Source: three-view drawing plus pictorial views. Frame: mm from the lowest corner of the part. Coordinates: 2 decimals unless noted, no trailing zeros. Write each loop counter-clockwise with the first axis right and the second up, starting at its lowest first coordinate (ties: lowest second). Pieces come first, ordered by that corner, then holes. Notation, with made-up numbers: (-33, -36) - (13, -36) arc R4 ccw to (13, -31) - close; hole circle Ø7 at (29, 72). An arc over 180 degrees is marked (long way). Put each result on its own line as item: value. Start each with the question number.
1. Pin query (flat end, axial travel): pin 1 (3 mm diameter, centred on y = 26.5, z = 4, fed in from -X); pin 2 (7 mm diameter, centred on x = 10, y = 10, fed in from -Z). Return the tip coordinate at first contact, or that it passes through.
2. Cut plane A-A, the plane y = 10. Return loops of the section in (x, z), and give its area (3 significant figures).
3. Cut plane D-D, the plane y = 25. Return loops of the section in (x, z).
4. Cut plane C-C, the plane x = 35. Return loops of the section in (y, z).
5. Pull-direction query (Y, two-part tool) for the marked faces 1, 2 and 3; classes: released by +Y, released by -Y, zero draft, split by the parting line, or undercut.
6. Cut plane B-B, the plane z = 5.25. Return loops of the section in (x, y).
7. Line query: line 1 (Y direction, x = 35, z = 3.8); line 2 (X direction, y = 7.5, z = 2); line 3 (Y direction, x = 35, z = 3.7). Output: solid intervals per line, ascending.
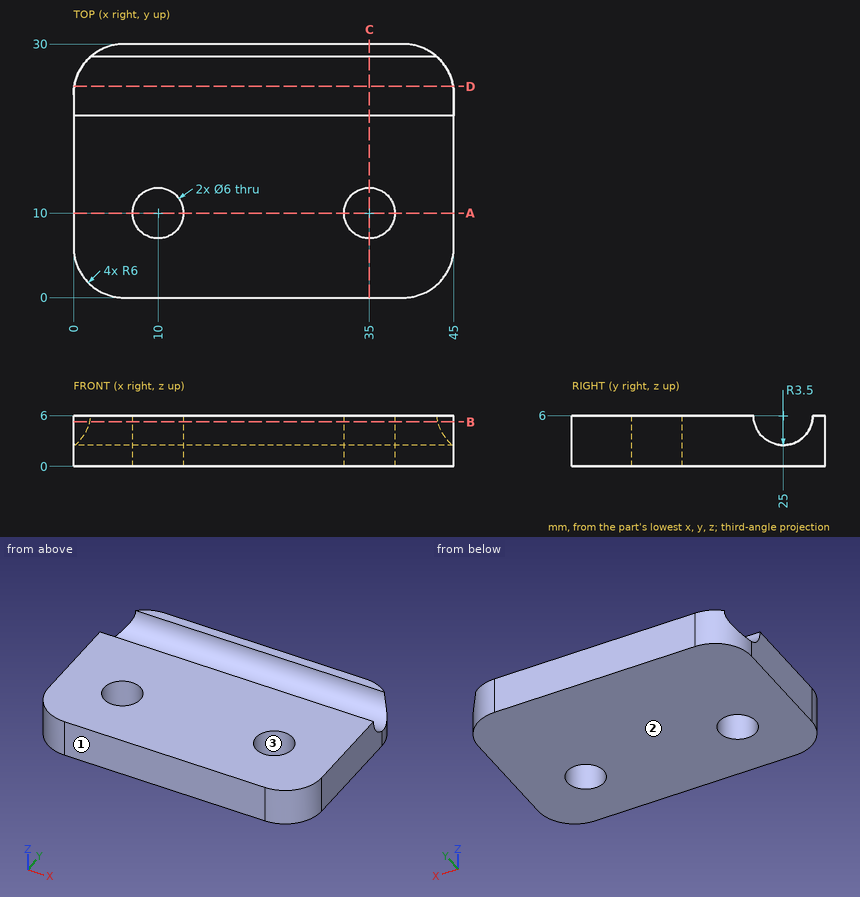
Report:
1. pin 1: stops at x = 0.31
1. pin 2: stops at z = 0
2. outline: (0, 0) - (7, 0) - (7, 6) - (0, 6) - close; (13, 0) - (32, 0) - (32, 6) - (13, 6) - close; (38, 0) - (45, 0) - (45, 6) - (38, 6) - close
2. area: 198 mm^2
3. outline: (0.08, 0) - (44.92, 0) - (44.92, 2.5) - (0.08, 2.5) - close
4. outline: (0, 0) - (7, 0) - (7, 6) - (0, 6) - close; (13, 0) - (30, 0) - (30, 6) - (28.5, 6) arc R3.5 cw to (21.5, 6) - (13, 6) - close
5. face 1: released by -Y
5. face 2: zero draft
5. face 3: undercut
6. outline: (0, 6) arc R6 ccw to (6, 0) - (39, 0) arc R6 ccw to (45, 6) - (45, 21.58) - (0, 21.58) - close; (1.94, 28.42) - (43.06, 28.42) arc R6 ccw to (39, 30) - (6, 30) arc R6 ccw to start; hole circle Ø6 at (10, 10); hole circle Ø6 at (35, 10)
7. line 1: y = 0 to 7, 13 to 22.28, 27.72 to 30
7. line 2: x = 0 to 8.34, 11.66 to 33.34, 36.66 to 45
7. line 3: y = 0 to 7, 13 to 22.36, 27.64 to 30
